Design review of the part built by this model. Coordinates are the model's own, in mm. A direction names the side the tool comes from. Give positions to 0.01 mm unless a question says otherwise; leave off trailing zeros. Loops run counter-clockwise (first coordinate to the right, second up) from the corner with the lowest first, then second, coordinate; pieces in that order, holes last.
from build123d import *

# Parameters (mm, degrees)
PCB_EXTRUDE_DEPTH            = 1
SKETCH3_R                    = 1.6
PCB_HOLES_AND_TABS_DEPTH     = 2
UART_EXTRUDE_DEPTH           = 5.5
SKETCH4_3_W                  = 3.8
SKETCH4_3_H                  = 7.3
BATTERY_AND_FAN_HEADER_DEPTH = 6
SKETCH4_4_W                  = 40.534718927
SKETCH4_4_H                  = 39.475094106
HEATSINK_FAN_DEPTH           = 14.7
SKETCH4_6_W                  = 6
SKETCH4_6_H                  = 6
POWERBUTTON_DEPTH            = 3.5
SKETCH5_R                    = 1.5
POWERBUTTONSWITCH_DEPTH      = 8.5
SKETCH4_8_W                  = 7.6
SKETCH4_8_H                  = 10.983605977
DCPOWERJACK_DEPTH            = 9.8
SKETCH4_11_R                 = 1.6
HEATSINKMOUNTTABS_DEPTH      = 2.25
SKETCH6_R                    = 2.5
HEATSINKSPRINGS_DEPTH        = 17.5
SKETCH4_13_W                 = 11.4
SKETCH4_13_H                 = 5.25
MICROSD_DEPTH                = 2.8
SKETCH7_R                    = 2.5
SKETCH7_W                    = 13.5
SKETCH7_H                    = 18.5
UNDERSIDE_DEPTH              = 4
GROSS_COMPONENTS_15_W        = 16
GROSS_COMPONENTS_15_H        = 21.5
ETHERNET_DEPTH               = 14.7
GROSS_COMPONENTS_16_W        = 15
GROSS_COMPONENTS_16_H        = 17.193227116
USBX2_DEPTH                  = 16.8
GROSS_COMPONENTS_17_W        = 7
GROSS_COMPONENTS_17_H        = 21.5
USBVERTICAL_DEPTH            = 14.7
GROSS_COMPONENTS_18_W        = 15
GROSS_COMPONENTS_18_H        = 11.350223911
HDMI_DEPTH                   = 6.5
GROSS_COMPONENTS_19_W        = 3.930498855
GROSS_COMPONENTS_19_H        = 9
DIP_DEPTH                    = 3.75
GROSS_COMPONENTS_21_W        = 37.3
GROSS_COMPONENTS_21_H        = 6
GROSS_COMPONENTS_21_W_2      = 6
GROSS_COMPONENTS_21_H_2      = 19.3
PINHEADERS_DEPTH             = 6.5


with BuildPart() as part:
    # Sketch1 → PCB Extrude (new body)
    with BuildSketch(Plane(origin=(0, 0, 0), x_dir=(1, 0, 0), z_dir=(0, 1, 0))):
        with BuildLine():
            Line((-38.5, -29.5), (38.5, -29.5))
            ThreePointArc((38.5, -29.5), (40.621320344, -28.621320344), (41.5, -26.5))
            Line((41.5, -26.5), (41.5, 26.5))
            ThreePointArc((41.5, 26.5), (40.621320344, 28.621320344), (38.5, 29.5))
            Line((38.5, 29.5), (-38.5, 29.5))
            ThreePointArc((-38.5, 29.5), (-40.621320344, 28.621320344), (-41.5, 26.5))
            Line((-41.5, 26.5), (-41.5, -26.5))
            ThreePointArc((-41.5, -26.5), (-40.621320344, -28.621320344), (-38.5, -29.5))
        make_face()
    extrude(amount=-PCB_EXTRUDE_DEPTH)

    # Sketch3 → PCB Holes and Tabs (cut, through all)
    with BuildSketch(Plane(origin=(0, 0, 0), x_dir=(1, 0, 0), z_dir=(0, 1, 0))):
        with Locations((-12.830824848, 12.70463972)):
            Circle(SKETCH3_R)
        with Locations((38.231306466, -7.222675777)):
            Circle(SKETCH3_R)
        with Locations((-38, 26)):
            Circle(SKETCH3_R)
        with Locations((38, 26)):
            Circle(SKETCH3_R)
        with Locations((38, -26)):
            Circle(SKETCH3_R)
        with Locations((-38, -26)):
            Circle(SKETCH3_R)
    extrude(amount=-PCB_HOLES_AND_TABS_DEPTH, mode=Mode.SUBTRACT)

    # Gross Components → UART Extrude (add)
    with BuildSketch(Plane(origin=(-30.681810048, 0, -29.297110237), x_dir=(1, 0, 0), z_dir=(0, 1, 0))):
        Polygon((-7.232403514, -8.562818523), (-10.818189952, -8.562818523), (-10.818189952, -20.762818523), (-5.818189952, -20.762818523), (-5.818189952, -9.977032085), align=None)
    extrude(amount=UART_EXTRUDE_DEPTH)

    # Sketch4_3 → Battery and Fan Header (add)
    with BuildSketch(Plane(origin=(-30.681810048, 0, -29.297110237), x_dir=(1, 0, 0), z_dir=(0, 1, 0))):
        with Locations((-8.918189952, -29.954934674)):
            Rectangle(SKETCH4_3_W, SKETCH4_3_H)
        with Locations((17.820043283, -33.259722768)):
            Rectangle(SKETCH4_3_W, SKETCH4_3_H)
    extrude(amount=BATTERY_AND_FAN_HEADER_DEPTH)

    # Sketch4_4 → HeatSink_Fan (add)
    with BuildSketch(Plane(origin=(-30.681810048, 0, -29.297110237), x_dir=(1, 0, 0), z_dir=(0, 1, 0))):
        with Locations((43.386588798, -27.066596392)):
            Rectangle(SKETCH4_4_W, SKETCH4_4_H)
    extrude(amount=HEATSINK_FAN_DEPTH)

    # Sketch4_6 → PowerButton (add)
    with BuildSketch(Plane(origin=(-30.681810048, 0, -29.297110237), x_dir=(1, 0, 0), z_dir=(0, 1, 0))):
        with Locations((18.444226135, -2.797110237)):
            Rectangle(SKETCH4_6_W, SKETCH4_6_H)
    extrude(amount=POWERBUTTON_DEPTH)

    # Sketch5 → PowerButtonSwitch (add)
    with BuildSketch(Plane(origin=(0, 3.5, 0), x_dir=(1, 0, 0), z_dir=(0, 1, 0))):
        with Locations((-12.237583913, 26.5)):
            Circle(SKETCH5_R)
    extrude(amount=POWERBUTTONSWITCH_DEPTH)

    # Sketch4_8 → DCPowerJack (add)
    with BuildSketch(Plane(origin=(-30.681810048, 0, -29.297110237), x_dir=(1, 0, 0), z_dir=(0, 1, 0))):
        with Locations((27.627643628, -53.305307249)):
            Rectangle(SKETCH4_8_W, SKETCH4_8_H)
    extrude(amount=DCPOWERJACK_DEPTH)

    # Sketch4_11 → HeatSinkMountTabs (add)
    with BuildSketch(Plane(origin=(-30.681810048, 0, -29.297110237), x_dir=(1, 0, 0), z_dir=(0, 1, 0))):
        with BuildLine():
            Line((63.653948261, -39.769786014), (68.913116514, -39.769786014))
            ThreePointArc((68.913116514, -39.769786014), (72.163116514, -36.519786014), (68.913116514, -33.269786014))
            Line((68.913116514, -33.269786014), (63.653948261, -33.269786014))
            Line((63.653948261, -33.269786014), (63.653948261, -39.769786014))
        make_face()
        with Locations((68.913116514, -36.519786014)):
            Circle(SKETCH4_11_R, mode=Mode.SUBTRACT)
        with BuildLine():
            Line((17.8509852, -19.842470517), (23.119229334, -19.842470517))
            Line((23.119229334, -19.842470517), (23.119229334, -13.342470517))
            Line((23.119229334, -13.342470517), (17.8509852, -13.342470517))
            ThreePointArc((17.8509852, -13.342470517), (14.6009852, -16.592470517), (17.8509852, -19.842470517))
        make_face()
        with Locations((17.8509852, -16.592470517)):
            Circle(SKETCH4_11_R, mode=Mode.SUBTRACT)
    extrude(amount=HEATSINKMOUNTTABS_DEPTH)

    # Sketch6 → HeatSinkSprings (add)
    with BuildSketch(Plane(origin=(0, 2.25, 0), x_dir=(1, 0, 0), z_dir=(0, 1, 0))):
        with Locations((38.231306466, -7.222675777)):
            Circle(SKETCH6_R)
        with Locations((-12.830824848, 12.70463972)):
            Circle(SKETCH6_R)
    extrude(amount=HEATSINKSPRINGS_DEPTH)

    # Sketch4_13 → microSD (add)
    with BuildSketch(Plane(origin=(-30.681810048, 0, -29.297110237), x_dir=(1, 0, 0), z_dir=(0, 1, 0))):
        with Locations((40.797038503, -51.062962156)):
            Rectangle(SKETCH4_13_W, SKETCH4_13_H)
    extrude(amount=MICROSD_DEPTH)

    # Sketch7 → UnderSide (add)
    with BuildSketch(Plane.XZ.offset(1)):
        with Locations((-12.830824848, -12.70463972)):
            Circle(SKETCH7_R)
        with Locations((38.231306466, 7.222675777)):
            Circle(SKETCH7_R)
        with Locations((10.25, 20.25)):
            Rectangle(SKETCH7_W, SKETCH7_H)
    extrude(amount=UNDERSIDE_DEPTH)

    # Gross Components_15 → Ethernet (add)
    with BuildSketch(Plane(origin=(-30.681810048, 0, -29.297110237), x_dir=(1, 0, 0), z_dir=(0, 1, 0))):
        with Locations((4.681810048, -48.047110237)):
            Rectangle(GROSS_COMPONENTS_15_W, GROSS_COMPONENTS_15_H)
    extrude(amount=ETHERNET_DEPTH)

    # Gross Components_16 → USBx2 (add)
    with BuildSketch(Plane(origin=(-30.681810048, 0, -29.297110237), x_dir=(1, 0, 0), z_dir=(0, 1, 0))):
        with Locations((4.981810048, -8.393723795)):
            Rectangle(GROSS_COMPONENTS_16_W, GROSS_COMPONENTS_16_H)
    extrude(amount=USBX2_DEPTH)

    # Gross Components_17 → USBvertical (add)
    with BuildSketch(Plane(origin=(-30.681810048, 0, -29.297110237), x_dir=(1, 0, 0), z_dir=(0, 1, 0))):
        with Locations((18.181810048, -48.047110237)):
            Rectangle(GROSS_COMPONENTS_17_W, GROSS_COMPONENTS_17_H)
    extrude(amount=USBVERTICAL_DEPTH)

    # Gross Components_18 → HDMI (add)
    with BuildSketch(Plane(origin=(-30.681810048, 0, -29.297110237), x_dir=(1, 0, 0), z_dir=(0, 1, 0))):
        with Locations((56.681810048, -53.121998282)):
            Rectangle(GROSS_COMPONENTS_18_W, GROSS_COMPONENTS_18_H)
    extrude(amount=HDMI_DEPTH)

    # Gross Components_19 → DIP (add)
    with BuildSketch(Plane(origin=(-30.681810048, 0, -29.297110237), x_dir=(1, 0, 0), z_dir=(0, 1, 0))):
        with Locations((70.216560621, -46.997110237)):
            Rectangle(GROSS_COMPONENTS_19_W, GROSS_COMPONENTS_19_H)
    extrude(amount=DIP_DEPTH)

    # Gross Components_21 → PinHeaders (add)
    with BuildSketch(Plane(origin=(-30.681810048, 0, -29.297110237), x_dir=(1, 0, 0), z_dir=(0, 1, 0))):
        with Locations((43.106667362, -4.197110237)):
            Rectangle(GROSS_COMPONENTS_21_W, GROSS_COMPONENTS_21_H)
        with Locations((68.181810048, -16.871799168)):
            Rectangle(GROSS_COMPONENTS_21_W_2, GROSS_COMPONENTS_21_H_2)
    extrude(amount=PINHEADERS_DEPTH)


solid = part.part
Q1. Tool access review of faces 1 (the face through (-12, 2, -23.5)), 2 (the face through (-18, 7, 19)), 3 (the face through (36, 1, 10.473)), 4 (the face through (-40, 3, -20.734)): name each direction out of +Z, -Z, +X, -X, +Y, -Y from which nothing blocks a thin tool from reaching the whole face with its end or side.
Results:
face 1: +Y
face 2: +Z, -Z, +Y
face 3: +X, +Y
face 4: -Z, -X, +Y
Q2. Take a section at D-D (x = -2). Give the boundary of the cut face in (y, z).
Results:
outline: (-1, -29.5) - (0, -29.5) - (0, -28.1) - (6.5, -28.1) - (6.5, -22.1) - (0, -22.1) - (0, -21.97) - (14.7, -21.97) - (14.7, 17.51) - (0, 17.51) - (0, 18.52) - (9.8, 18.52) - (9.8, 29.5) - (-1, 29.5) - close
Q3. Take a section at C-C (y = 18.25). Give the boundary of the cut face in (x, z), plus the area to 3 significant figures.
Results:
outline: circle Ø5 at (-12.83, -12.7); circle Ø5 at (38.23, 7.22)
area: 39.3 mm2
Q4. Insertion check: pin 1 (2 mm diameter, centred on x = 22.5, y = 7, fed in from -Z); pin 2 (1 mm diameter, centred on y = 7, z = -18.5, fed in from -X); pin 3 (4 mm diameter, centred on x = -38, y = 3, fed in from +Z). Each pin has a flat end and moves straight along its axis. Give the tip position at first contact, or say it passes through.
Results:
pin 1: stops at z = -28.1
pin 2: stops at x = -33.2
pin 3: stops at z = 4.31
Q5. Take a section at A-A (x = -22.5). Give the boundary of the cut face in (y, z).
Results:
outline: (-1, -29.5) - (16.8, -29.5) - (16.8, -12.31) - (0, -12.31) - (0, 8) - (14.7, 8) - (14.7, 29.5) - (-1, 29.5) - close
Q6. Wall thickness on line 1 (X direction, y = -0.65, z = -26); line 2 (X direction, y = 8, z = 11.5); line 3 (Z direction, x = -13, y = 1): over which ranges is each line inside the solid? List them lowest first.
Results:
line 1: x = -41.5 to -39.6, -36.4 to 36.4, 39.6 to 41.5
line 2: x = -34 to -18, -16 to -9, -7.56 to 32.97
line 3: z = -29.5 to -23.5, -15.95 to -14.3, -11.11 to -9.46, 0.31 to 7.61, 8 to 29.5
Q7. Draft analysis for pull direction X (two halves, no side actions). For faces 5 (the face through (-37.7, 3, 1)), 6 (the face through (37, 6.5, -13)), 7 (the face through (-14.81, -2.97, -14.23)), state which applies: pulls with the +X half, pulls with the -X half, needs draft (parallel to the pull), parting line crosses it, or undercut.
Results:
face 5: undercut
face 6: needs draft
face 7: parting line crosses it
